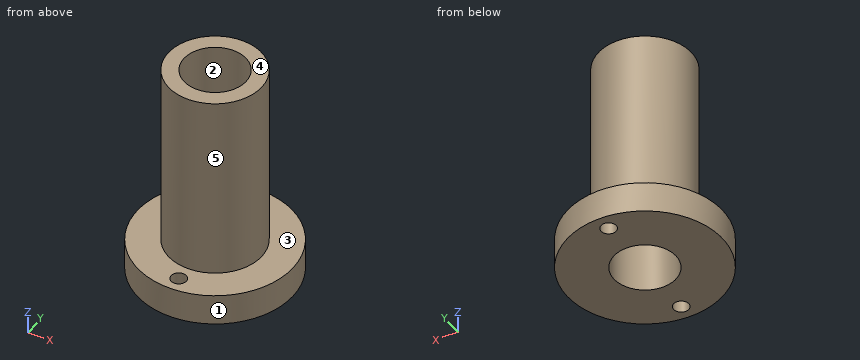
Autodesk Inventor part; units mm, degrees
ref_plane "YZ Plane" through (0, 0, 0) normal (1, 0, 0) x (0, 1, 0)
ref_plane "XZ Plane" through (0, 0, 0) normal (0, 1, 0) x (-1, 0, 0)
ref_plane "XY Plane" through (0, 0, 0) normal (0, 0, 1) x (1, 0, 0)
sketch "スケッチ1" plane through (0, 0, 0) normal (0, 0, 1) x (1, 0, 0)
  circle A0 centre (0, 0) radius 12.5
  dimension "d0" = 25
extrude "押し出し1" add sketch "スケッチ1" along normal blind 5
sketch "スケッチ2" plane through (0, 0, 5) normal (0, 0, 1) x (1, 0, 0)
  circle A0 centre (0, 0) radius 7.5
  dimension "d3" = 15
extrude "押し出し2" add sketch "スケッチ2" along normal blind 30
sketch "スケッチ3" plane through (0, 0, 0) normal (0, 0, -1) x (-1, 0, 0)
  circle A0 centre (0, 0) radius 5
  dimension "d6" = 10
extrude "押し出し3" cut sketch "スケッチ3" against normal blind 35
sketch "スケッチ4" plane through (0, 0, 5) normal (0, 0, 1) x (1, 0, 0)
  line L0 (0, 0) -> (-12.5, 0) construction
  circle A0 centre (0, 0) radius 12.5
  point P0 (0, -10)
  point P1 (0, 10)
  dimension "d9" = 20
hole "穴1" at (0, -10, 5) at (0, 10, 5) direction (0, 0, -1) diameter 2.459 end through all
properties part number "RD005_ペンホルダ"
Source: CAD feature listing. Evaluate the final solid. Frame: model axes, mm. Face numbers are marked on the shaded views. A direction names the side the tool comes from. Round coordinates to 2 decimals unless told otherwise and drop trailing zeros. Write each loop counter-clockwise with the first axis right and the second up, starting at its lowest first coordinate (ties: lowest second). Pieces come first, ordered by that corner, then holes. Notation, with made-up numbers: (20.5, 59.5) - (34.5, 59.5) arc R27 cw to (34.5, 98.5) - close; hole circle Ø9 at (49, 8). An arc over 180 degrees is marked (long way). Use CSV: the item, a comma, the result in double quotes. Start each with the question number.
(1) Mould query, pull axis Y, two halves, no side actions, for the marked faces 1, 2 and 3. Classes: pulls with the +Y half, pulls with the -Y half, needs draft (parallel to the pull), parting line crosses it, or undercut.
(2) Cut plane A-A, the plane y = 0. Return loops of the section in (x, z), and give its area (3 significant figures).
(3) Cut plane B-B, the plane x = 0. Return loops of the section in (y, z), and give its area (3 significant figures).
(4) Cut plane C-C, the plane z = 10. Return loops of the section in (x, y), and give its area (3 significant figures).
(5) Material intervals for probe 1 along Y at (x, z) = (0, 2.05); probe 2 along X at (y, z) = (10, 3.25); probe 3 along Y at (x, z) = (0, 12), sorted ascending. Write a range as [from, to].
(6) Cut plane D-D, the plane y = -10. Return loops of the section in (x, z), and give its area (3 significant figures).
(7) Set-up query: the marked faces 4 and 5. Return all of +Z, -Z, +X, -X, +Y, -Y with unobstructed straight access to the full face (end or side cutting, diameter ignored); none if empty.
(8) First-contact query: pin 1 Ø5 at (y, z) = (0.5, 24) entering from -X; pin 2 Ø8 at (x, z) = (4, 27.5) entering from -Y; pin 3 Ø12 at (y, z) = (9.5, 29) entering from -X. Flat tips, straight axial feed; report the tip coordinate or a pass-through.
Geometry says:
1,face 1,"parting line crosses it"
1,face 2,"undercut"
1,face 3,"needs draft"
2,outline,"(-12.5, 0) - (-5, 0) - (-5, 35) - (-7.5, 35) - (-7.5, 5) - (-12.5, 5) - close; (5, 0) - (12.5, 0) - (12.5, 5) - (7.5, 5) - (7.5, 35) - (5, 35) - close"
2,area,"225 mm²"
3,outline,"(-12.5, 0) - (-11.23, 0) - (-11.23, 5) - (-12.5, 5) - close; (-8.77, 0) - (-5, 0) - (-5, 35) - (-7.5, 35) - (-7.5, 5) - (-8.77, 5) - close; (5, 0) - (8.77, 0) - (8.77, 5) - (7.5, 5) - (7.5, 35) - (5, 35) - close; (11.23, 0) - (12.5, 0) - (12.5, 5) - (11.23, 5) - close"
3,area,"200 mm²"
4,outline,"circle Ø15 at (0, 0); hole circle Ø10 at (0, 0)"
4,area,"98.2 mm²"
5,probe 1,"[-12.5, -11.23], [-8.77, -5], [5, 8.77], [11.23, 12.5]"
5,probe 2,"[-7.5, -1.23], [1.23, 7.5]"
5,probe 3,"[-7.5, -5], [5, 7.5]"
6,outline,"(-7.5, 0) - (-1.23, 0) - (-1.23, 5) - (-7.5, 5) - close; (1.23, 0) - (7.5, 0) - (7.5, 5) - (1.23, 5) - close"
6,area,"62.7 mm²"
7,face 4,"+Z, +X, -X, +Y, -Y"
7,face 5,"+Z"
8,pin 1,"x = -7.5"
8,pin 2,"y = -7.5"
8,pin 3,"x = -6.63"
